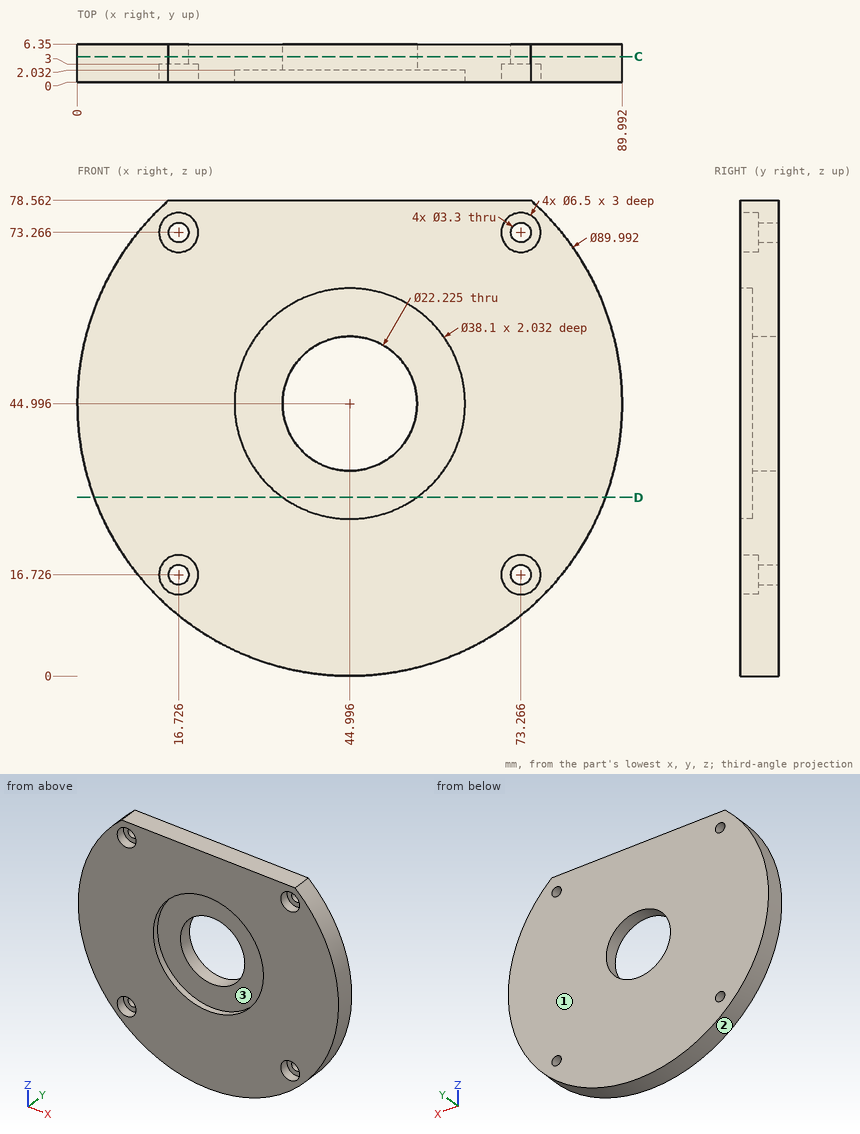
Check sheet for the drawn part. Datum: minimum x, y, z corner. Units: mm. Give positions to 0.01 mm unless a question says otherwise; leave off trailing zeros. Order: outer loops, then holes, each group sorted by start corner. A loop starts at its lowest first (then second) coordinate and runs counter-clockwise, first axis right, second up. Notation, with made-up numbers: (10.25, 81.25) -> (56.25, 81.25) arc R21 ccw to (56.25, 96.25) -> close; hole circle Ø9 at (55.5, 11.25). An arc over 180 degrees is marked (long way). Use a Markdown table: item, result.
1) Material ranges on probe 1 along X at (y, z) = (1.75, 16) (1 decimal); probe 2 along Z at (x, y) = (72.5, 5.25) (1 decimal); probe 3 along Z at (x, y) = (22, 4.75), recorded low to high.
Results:
| item | result |
|---|---|
| probe 1 | 10.6 to 13.6, 19.9 to 70.1, 76.4 to 79.4 |
| probe 2 | 9.4 to 15.3, 18.2 to 71.8, 74.7 to 78.6 |
| probe 3 | 6.32 to 78.56 |
2) Section check C-C, the plane y = 4.25. Give the number of separate pieces and of enclosed holes in the cut face, then the cut area to 3 significant figures.
Results:
| item | result |
|---|---|
| separate pieces | 1 |
| enclosed holes | 5 |
| area | 5,470 mm² |
3) Section check D-D, the plane z = 29.5. Record the boundary of the cut face in (x, y).
Results:
| item | result |
|---|---|
| outline | (2.75, 0) -> (33.92, 0) -> (33.92, 2.03) -> (56.08, 2.03) -> (56.08, 0) -> (87.24, 0) -> (87.24, 6.35) -> (2.75, 6.35) -> close |
4) Depth check by flat-ended pin: pin 1 Ø2 at (y, z) = (4, 19.5) entering from +X; pin 2 Ø2 at (x, z) = (16.5, 72) entering from -Y; pin 3 Ø1.5 at (x, z) = (58, 42) entering from -Y. Enter the tip coordinate at first touch or a pass-through.
Results:
| item | result |
|---|---|
| pin 1 | x = 82.74 |
| pin 2 | y = 3 |
| pin 3 | y = 2.03 |
5) Mould release check, pull along X, two halves, no side actions. Record for the marked faces 1, 2 and 3: pulls with the +X half, pulls with the -X half, needs draft (parallel to the pull), parting line crosses it, or undercut.
Results:
| item | result |
|---|---|
| face 1 | needs draft |
| face 2 | parting line crosses it |
| face 3 | undercut |
